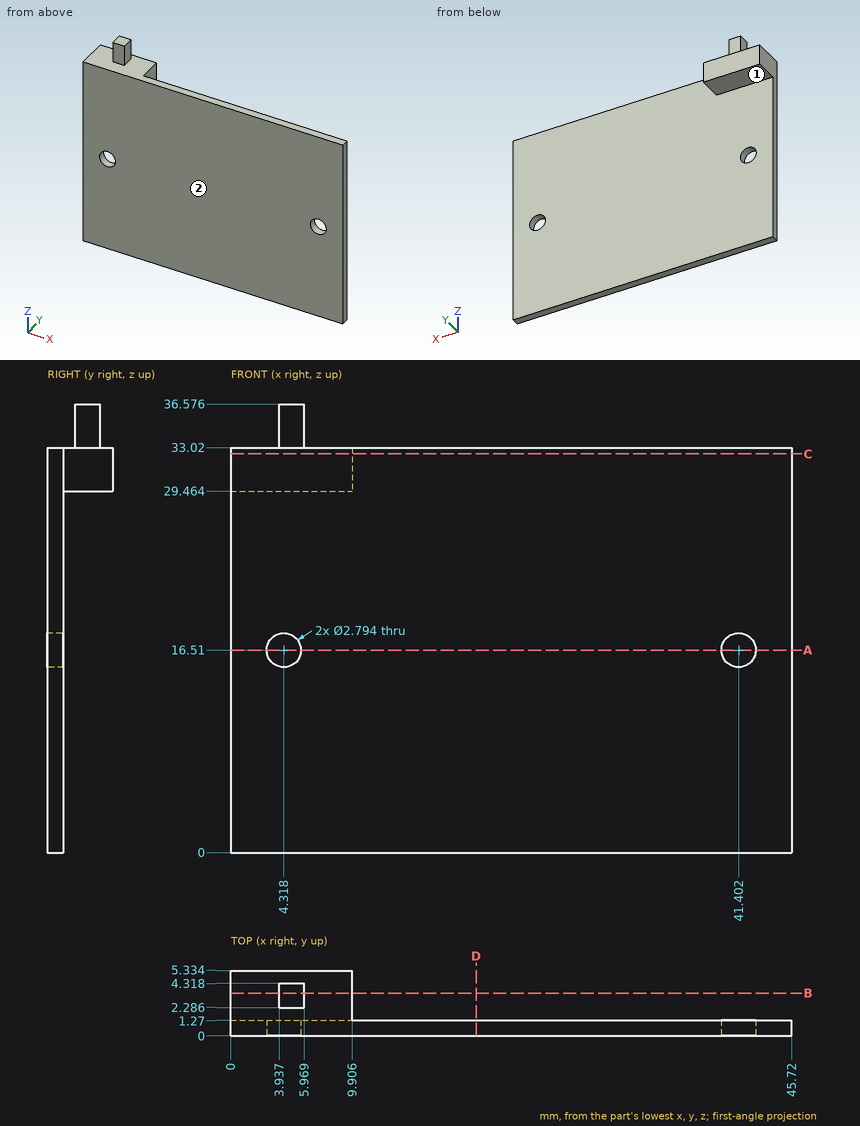
Geometry check sheet. Reference: drawing and pictorial views, mm from the part's lowest x, y, z. A direction names the side the tool comes from. Give positions to 0.01 mm unless a question says otherwise; leave off trailing zeros. Write each loop counter-clockwise with the first axis right and the second up, starting at its lowest first coordinate (ties: lowest second). Pieces come first, ordered by that corner, then holes. Notation, with made-up numbers: (9.5, -15) -> (25.5, -15) arc R17 cw to (25.5, 6) -> close; hole circle Ø5 at (-39.5, 22). An arc over 180 degrees is marked (long way). One line per item, written item: value. Start each with the question number.
Item 1: Section check C-C on z = 32.5. Record the cut outline in (x, y), then the cut area to 3 significant figures.
Item 2: Section check A-A on z = 16.51. Record the cut outline in (x, y) (3 decimals).
Item 3: Tool access check on the marked faces 1 and 2. Record the directions out of +Z, -Z, +X, -X, +Y, -Y that give a thin tool (end or side, any length) a straight path to the whole face; none if there is none.
Item 4: Gauge pin test, flat ends, axial feed: pin 1 (2 mm diameter, centred on y = 1.5, z = 14.5, fed in from +X); pin 2 (1 mm diameter, centred on x = 5, z = 34, fed in from +Y); pin 3 (2.5 mm diameter, centred on x = 41.402, z = 16.51, fed in from -Y); pin 4 (1.6 mm diameter, centred on x = 5, z = 35, fed in from -Y). Record the tip position at first contact, or that the pin passes through.
Item 5: Section check B-B on y = 3.5. Record the cut outline in (x, z).
Item 6: Section check D-D on x = 20. Record the cut outline in (y, z).
Item 7: Material ranges on probe 1 along X at (y, z) = (0.45, 16.51) (3 decimals); probe 2 along Z at (x, y) = (7, 2.4); probe 3 along Z at (x, y) = (37, 1.15), recorded low to high. Write a range as from..to.
Results list:
1. outline: (0, 0) -> (45.72, 0) -> (45.72, 1.27) -> (9.91, 1.27) -> (9.91, 5.33) -> (0, 5.33) -> close
1. area: 98.3 mm²
2. outline: (0, 0) -> (2.921, 0) -> (2.921, 1.27) -> (0, 1.27) -> close; (5.715, 0) -> (40.005, 0) -> (40.005, 1.27) -> (5.715, 1.27) -> close; (42.799, 0) -> (45.72, 0) -> (45.72, 1.27) -> (42.799, 1.27) -> close
3. face 1: -Z, +X, -X, +Y
3. face 2: +Z, -Z, +X, -X, -Y
4. pin 1: x = 45.72
4. pin 2: y = 4.32
4. pin 3: through
4. pin 4: y = 2.29
5. outline: (0, 29.46) -> (9.91, 29.46) -> (9.91, 33.02) -> (5.97, 33.02) -> (5.97, 36.58) -> (3.94, 36.58) -> (3.94, 33.02) -> (0, 33.02) -> close
6. outline: (0, 0) -> (1.27, 0) -> (1.27, 33.02) -> (0, 33.02) -> close
7. probe 1: 0..2.921, 5.715..40.005, 42.799..45.72
7. probe 2: 29.46..33.02
7. probe 3: 0..33.02
